Autodesk Inventor part; units mm, degrees
ref_plane "YZ Plane" through (0, 0, 0) normal (1, 0, 0) x (0, 1, 0)
ref_plane "XZ Plane" through (0, 0, 0) normal (0, 1, 0) x (-1, 0, 0)
ref_plane "XY Plane" through (0, 0, 0) normal (0, 0, 1) x (1, 0, 0)
sketch "Sketch1" plane through (0, 0, 0) normal (1, 0, 0) x (0, 1, 0)
  line L0 (0, 0) -> (25.4, 0)
  line L1 (25.4, 0) -> (25.4, -9.525)
  line L2 (25.4, -9.525) -> (0, -9.525)
  line L3 (0, -9.525) -> (0, 0)
  line L4 (25.4, -9.525) -> (35.5298, -9.525)
  line L5 (35.5298, -9.525) -> (35.5298, -29.845)
  line L6 (25.4, -9.525) -> (25.4, -24.4288)
  line L7 (25.4, -24.4288) -> (25.4, -29.845)
  line L8 (35.5298, -29.845) -> (26.0048, -29.845)
  line L9 (26.0048, -29.845) -> (26.0048, -80.645)
  line L10 (26.0048, -80.645) -> (35.5298, -80.645)
  line L11 (35.5298, -80.645) -> (35.5298, -29.845)
  line L12 (35.5298, -80.645) -> (41.8798, -80.645)
  line L13 (41.8798, -80.645) -> (41.8798, -15.4958)
  line L14 (41.8798, -15.4958) -> (35.5298, -15.4958)
  line L15 (35.5298, -15.4958) -> (35.5298, -80.645)
  line L16 (25.4, 0) -> (35.5298, -9.525)
  line L17 (41.8798, -15.4958) -> (35.5298, -9.525)
  line L18 (26.0048, -29.845) -> (25.4, -29.845)
  line L19 (0, 0) -> (-76.2, 0)
  line L20 (-76.2, 0) -> (-76.2, -9.525)
  line L21 (-76.2, -9.525) -> (0, -9.525)
  line L22 (0, -9.525) -> (0, 0)
  dimension "d0" = 25.4
  dimension "d1" = 9.525
  dimension "d3" = 20.32
  dimension "d11" = 50.8
  dimension "d12" = 6.35
  dimension "d13" = 76.2
  dimension "d14" = 9.525
extrude "Extrusion1" add sketch "Sketch1" along normal blind 19.05
sketch "Sketch4" plane through (0, 26.0048, -80.645) normal (0, -1, 0) x (1, 0, 0)
  line L0 (0, 0) -> (0, 65.1492)
  line L1 (19.05, 71.12) -> (19.05, 50.8)
  line L2 (0, 0) -> (19.05, 0)
  line L3 (19.05, 0) -> (19.05, 71.12)
  line L4 (19.05, 71.12) -> (0, 71.12)
  line L5 (0, 71.12) -> (0, 0)
  point P0 (0, 80.645)
  point P1 (0, 65.1492)
extrude "Extrusion3" add sketch "Sketch4" along normal blind 16.256
sketch "Sketch5" plane through (0, 41.8798, -15.4958) normal (0, 1, 0) x (1, 0, 0)
  line L0 (0, 65.1492) -> (19.05, 65.1492)
  line L1 (0, 0) -> (19.05, 0)
  line L2 (0, 65.1492) -> (12.7, 65.1492)
  line L3 (12.7, 65.1492) -> (12.7, 0)
  line L4 (12.7, 0) -> (0, 0)
  line L5 (0, 0) -> (0, 65.1492)
  point P0 (0, -15.4958)
  dimension "d17" = 12.7
extrude "Extrusion4" cut sketch "Sketch5" against normal blind 9.525
sketch "Sketch6" plane through (0, 0, 0) normal (-1, 0, 0) x (0, 0, 1)
  circle A0 centre (-20.3035, 23.5915) radius 1.7907
  point P0 (0, 0)
  dimension "d20" = 3.5814
extrude "Extrusion5" cut sketch "Sketch6" against normal blind 92.075
sketch "Sketch7" plane through (0, -76.2, 0) normal (0, 0, 1) x (1, 0, 0)
  line L0 (0, 0) -> (19.05, 0)
  line L1 (0, 0) -> (19.05, 0)
  line L2 (19.05, 0) -> (19.05, 19.05)
  line L3 (19.05, 19.05) -> (0, 19.05)
  line L4 (0, 19.05) -> (0, 0)
  point P0 (0, 76.2)
  dimension "d23" = 19.05
  dimension "d24" = 19.05
extrude "Extrusion6" add sketch "Sketch7" along normal blind 19.05
sketch "Sketch8" plane through (0, 0, 0) normal (-1, 0, 0) x (0, 0, 1)
  line L0 (-9.525, -76.2) -> (19.05, -76.2)
  line L1 (0, -57.15) -> (19.05, -76.2)
  line L2 (19.05, -76.2) -> (19.05, -57.15)
  line L3 (19.05, -57.15) -> (0, -76.2)
  circle A0 centre (9.525, -66.675) radius 1.7907
  point P0 (0, 0)
  dimension "d27" = 3.5814
extrude "Extrusion7" cut sketch "Sketch8" against normal blind 31.75 contours A0 L1 L3 | L3 L1 A0 | L1 L3 A0 | L1 A0 L3
properties part number "GripperServoAtt"
Could you check a few things on this model? Use its own coordinates, in mm. A direction names the side the tool comes from. Coordinates: 2 decimals unless noted, no trailing zeros. Loops run counter-clockwise (first coordinate to the right, second up) from the corner with the lowest first, then second, coordinate; pieces in that order, holes last. Notation, with made-up numbers: M -3.5,-21 L 6.5,-21 A15 ccw 6.5,-17 Z; hole C -10,62.5 d3. An arc over 180 degrees is marked long. Put each result on its own line as item: value. Start each with the question number.
(1) Will these pins go through, and if not, where does the flat tip stop? P1, Ø9.5, axis at x = 6, z = -28, coming from the -Y side; P2, Ø3, axis at x = 11, y = -46.5, coming from the -Z side (3 decimals); P3, Ø1, axis at x = 7, z = -36, coming from the +Y side.
(2) Suppose I cut it at B-B on z = -71.5. Please give me the cut outline in (x, y).
(3) Thinking about a two-plate mould opening in Y: for faces 4 (the face through (0, -4, -9)), 5 (the face through (9.392, -68.264, 10.351)), 6 (the face through (10, -57.15, 9)), which applies, pulls with the +Y half, pulls with the -Y half, needs draft (parallel to the pull), parting line crosses it, or undercut?
(4) I need wall thicknesses on line 1 (Y direction, x = 8.5, z = 9.5); line 2 (Z direction, x = 8, y = -27) (3 decimals); line 3 (Y direction, x = 13.25, z = 3). Which ranges of each line are inside material? Lowest first, please. Write a range as from..to.
(5) Suppose I cut it at C-C on y = 19. Please give me the cut outline in (x, z) (3 decimals), then the cut area to 3 significant figures.
(6) Suppose I cut it at A-A on x = 17.5. Count the separate pieces of the cut face and the enclosed holes in it, then the cut area to 3 significant figures.
(7) For faces 1 (the face through (6, 37, -15.496)), 2 (the face through (9, -33, -9.525)), 3 (the face through (9, -16, 0)), which set-ups out of +Z, -Z, +X, -X, +Y, -Y let a thin tool reach every point of the face, with its end or its side?
Solutions:
1. P1: stops at y = 9.75
1. P2: stops at z = -9.525
1. P3: stops at y = 32.35
2. outline: M 0,9.75 L 19.05,9.75 L 19.05,41.88 L 12.7,41.88 L 12.7,32.35 L 0,32.35 Z
3. face 4: needs draft
3. face 5: undercut
3. face 6: pulls with the +Y half
4. line 1: y = -76.2..-68.47, -64.88..-57.15
4. line 2: z = -9.525..0
4. line 3: y = -76.2..-57.15
5. outline: M 0,-80.645 L 19.05,-80.645 L 19.05,0 L 0,0 Z
5. area: 1,540 mm2
6. separate pieces: 1
6. enclosed holes: 2
6. area: 3,620 mm2
7. face 1: -Z, -X, +Y
7. face 2: -Z, +X, -X, -Y
7. face 3: +Z, +X, -X, +Y
